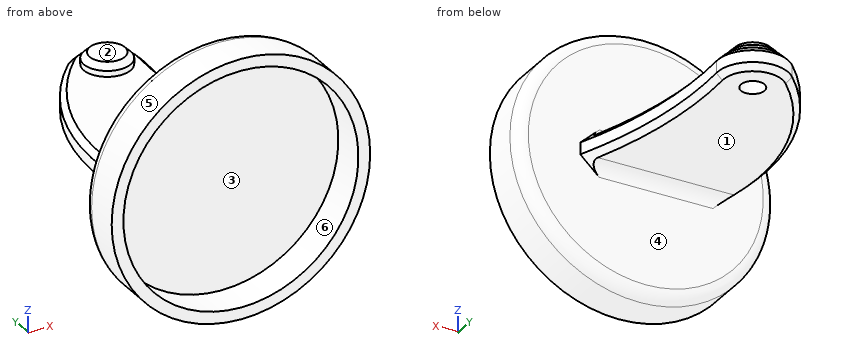
from build123d import *

# Parameters (mm, degrees)
SKETCH2_R           = 55
BOSS_EXTRUDE1_DEPTH = 20
FILLET1_R           = 5
BOSS_EXTRUDE2_DEPTH = 5
CHAMFER1_SIZE       = 2.5
CHAMFER2_SIZE       = 2.5
FILLET2_R           = 5
SKETCH4_R           = 10
BOSS_EXTRUDE3_DEPTH = 5
CHAMFER3_SIZE       = 2.5
SKETCH5_R           = 5
CUT_EXTRUDE1_DEPTH  = 10
SKETCH8_R           = 50
CUT_EXTRUDE2_DEPTH  = 15


with BuildPart() as part:
    # Sketch2 → Boss-Extrude1 (new body)
    with BuildSketch(Plane(origin=(0, 0, 0), x_dir=(1, 0, 0), z_dir=(0, 1, 0))):
        with Locations(Location((0, 0, 0), (0, 0, 270))):
            Circle(SKETCH2_R)
    extrude(amount=BOSS_EXTRUDE1_DEPTH)

    # Fillet1
    fillet1_edges = [part.edges().sort_by_distance(p)[0] for p in [
        (0, 20, -55),
    ]]
    fillet(fillet1_edges, radius=FILLET1_R)

    # Sketch3 → Boss-Extrude2 (add, symmetric)
    with BuildSketch(Plane.XY):
        with BuildLine():
            Line((-35, 15), (30, 15))
            ThreePointArc((30, 15), (17.428098582, 56.126843631), (14.970645506, 99.06203778))
            ThreePointArc((14.970645506, 99.06203778), (6.012327577, 113.742340307), (-10.849201429, 110.358321696))
            ThreePointArc((-10.849201429, 110.358321696), (-35.460543036, 65.854059614), (-35, 15))
        make_face()
    extrude(amount=BOSS_EXTRUDE2_DEPTH, both=True)

    # Chamfer1
    chamfer1_edges = [part.edges().sort_by_distance(p)[0] for p in [
        (16.970295051, 58.803839559, 5),
        (6.012327577, 113.742340307, 5),
        (-34.796467261, 68.341174934, 5),
    ]]
    chamfer(chamfer1_edges, length=CHAMFER1_SIZE)

    # Chamfer2
    chamfer2_edges = [part.edges().sort_by_distance(p)[0] for p in [
        (-34.796467261, 68.341174934, -5),
        (16.970295051, 58.803839559, -5),
        (6.012327577, 113.742340307, -5),
    ]]
    chamfer(chamfer2_edges, length=CHAMFER2_SIZE)

    # Fillet2
    fillet2_edges = [part.edges().sort_by_distance(p)[0] for p in [
        (-4.241511046, 20, 5),
        (-4.241511046, 20, -5),
    ]]
    fillet(fillet2_edges, radius=FILLET2_R)

    # Sketch4 → Boss-Extrude3 (add)
    with BuildSketch(Plane.XY.offset(5)):
        with Locations(Location((0, 100, 0), (0, 0, 180))):
            Circle(SKETCH4_R)
    extrude(amount=BOSS_EXTRUDE3_DEPTH)

    # Chamfer3
    chamfer3_edges = [part.edges().sort_by_distance(p)[0] for p in [
        (10, 100, 10),
    ]]
    chamfer(chamfer3_edges, length=CHAMFER3_SIZE)

    # Sketch5 → Cut-Extrude1 (cut)
    with BuildSketch(Plane(origin=(0, 0, -5), x_dir=(-1, 0, 0), z_dir=(0, 0, -1))):
        with Locations((0, 100)):
            Circle(SKETCH5_R)
    extrude(amount=-CUT_EXTRUDE1_DEPTH, mode=Mode.SUBTRACT)

    # Sketch8 → Cut-Extrude2 (cut)
    with BuildSketch(Plane.XZ):
        with Locations(Location((0, 0, 0), (0, 0, 270))):
            Circle(SKETCH8_R)
    extrude(amount=-CUT_EXTRUDE2_DEPTH, mode=Mode.SUBTRACT)


solid = part.part
Input: part model. Units: mm. Frame: model coordinates. Face numbers are marked on the shaded views. A direction names the side the tool comes from. Coordinates: 2 decimals unless noted, no trailing zeros. Order: outer loops, then holes, each group sorted by start corner. A loop starts at its lowest first (then second) coordinate and runs counter-clockwise, first axis right, second up. Notation, with made-up numbers: M -21,-32 L -2,-32 A21 ccw -2,7 Z; hole C 26.5,15.25 d3. An arc over 180 degrees is marked long. Write item = value, one per line. Start each with the question number.
(1) First-contact query: P1, Ø10, axis at y = 20, z = 24, coming from the +X side; P2, Ø1, axis at x = 15, y = 19, coming from the +Z side; P3, Ø12, axis at y = 81.5, z = 10.5, coming from the -X side. Flat tips, straight axial feed; report the tip coordinate or a pass-through.
(2) Pull-direction query (X, two-part tool) for the marked faces 4, 5 and 6; classes: released by +X, released by -X, zero draft, split by the parting line, or undercut.
(3) Section C-C on y = 13. Output: boundary loops of the cut face in (x, z).
(4) Section B-B on x = 0. Output: boundary loops of the cut face in (y, z), and give its area (3 significant figures).
(5) Reachability of the marked faces 1, 2 and 3 from +Z, -Z, +X, -X, +Y, -Y: full face, straight path, thin tool, end or side. Return the list, or none.
(6) Section A-A on z = 0. Output: boundary loops of the cut face in (x, y), and give its area (3 significant figures).
(7) Line query: line 1 along Y through (x, z) = (0, -2); line 2 along X through (y, z) = (10, 0); line 3 along Y through (x, z) = (-40.5, 21.5). Output: solid intervals per line, ascending. Write a range as [from, to].
Result set:
q1.P1 = 50.82
q1.P2 = 51.45
q1.P3 = -28.4
q2.face_4 = zero draft
q2.face_5 = split by the parting line
q2.face_6 = undercut
q3.outline = C 0,0 d110; hole C 0,0 d100
q4.outline = M 0,-55 L 15,-55 A5 ccw 20,-50 L 20,-10 A5 cw 25,-5 L 95,-5 L 95,5 L 105,5 L 105,-5 L 112.5,-5 L 115,-2.5 L 115,2.5 L 112.5,5 L 110,5 L 110,7.5 L 107.5,10 L 92.5,10 L 90,7.5 L 90,5 L 25,5 A5 cw 20,10 L 20,50 A5 ccw 15,55 L 0,55 L 0,50 L 15,50 L 15,-50 L 0,-50 Z
q4.area = 1,640 mm²
q5.face_1 = -Z, +X, -X, +Y
q5.face_2 = +Z, +X, -X, +Y
q5.face_3 = -Y
q6.outline = M -55,0 L -50,0 L -50,15 L 50,15 L 50,0 L 55,0 L 55,15 A5 ccw 50,20 L 27.88,20 A180 cw 14.97,99.06 A15 ccw -10.85,110.36 A100 ccw -36.23,20 L -50,20 A5 ccw -55,15 Z; hole C 0,100 d10
q6.area = 5,160 mm²
q7.line_1 = [15, 95], [105, 115]
q7.line_2 = [-55, -50], [50, 55]
q7.line_3 = [15, 20]
